Model file for the job. Use its own axes, mm. A direction names the side the tool comes from. Coordinates: 2 decimals unless noted, no trailing zeros. Order: outer loops, then holes, each group sorted by start corner. A loop starts at its lowest first (then second) coordinate and runs counter-clockwise, first axis right, second up. Notation, with made-up numbers: (41, 38) -> (63, 38) arc R27 cw to (63, 60) -> close; hole circle Ø10 at (42, 89.5). An arc over 180 degrees is marked (long way). Return JSON: item names as keys, results as strings. Group by question number.
1) Cut at D-D (x = -10). Write the cut outline in (y, z), and give its area (3 significant figures).
2) Probe line 1 (Y direction, x = 0, z = -1); line 2 (Y direction, x = 27.5, z = -1); line 3 (Y direction, x = 18.5, z = 3.5). List the from-to ranges inside material, lowest first.
3) Which spindle directions (+Z, -Z, +X, -X, +Y, -Y) get a long thin tool onto all of the face, cutting with end or side? Do faces 4 (the conical face through (-0.17, -4.13, -5.69)), 5 (the flat face through (0, 4.8, 0)). Say none if no direction does.
4) Cut at A-A (x = 0). Write the cut outline in (y, z).
5) Cut at B-B (z = 1.5). Write the cut outline in (x, y), and give its area (3 significant figures).
6) Pull direction Y, two halves, no side cores. Call faces 1 (the conical face through (-0.17, -4.12, 5.68)), 2 (the cylindrical face through (-6.607, -29.755, 0.089)), 3 (the flat face through (6, 0, -6.35)): +Y half, -Y half, draft (parallel to the pull), parting line (faces both ways), or undercut.
7) Cut at C-C (y = 0). Write the cut outline in (x, z), and give its area (3 significant figures).
8) Flat gauge pins, fed straight in: pin 1 (2 mm diameter, centred on x = 0.5, z = -3, fed in from -Y); pin 2 (2 mm diameter, centred on x = 8, z = -1, fed in from +Y); pin 3 (5 mm diameter, centred on y = 12, z = 5, fed in from +X). Where does each tip first touch, or does it go through?
from build123d import *

# Parameters (mm, degrees)
SKETCH1_R          = 30.48
SKETCH1_R_2        = 4
EXTRUDE1_DEPTH     = 6.35
CHAMFER1_SIZE      = 0.79375
SKETCH3_W          = 2
SKETCH3_H          = 2
CUT_EXTRUDE1_DEPTH = 45.937187273


with BuildPart() as part:
    # Sketch1 → Extrude1 (new, symmetric)
    with BuildSketch(Plane.XY):
        Circle(SKETCH1_R)
        Circle(SKETCH1_R_2, mode=Mode.SUBTRACT)
    extrude(amount=EXTRUDE1_DEPTH, both=True)

    # Chamfer1
    chamfer1_edges = [part.edges().sort_by_distance(p)[0] for p in [
        (-4, 0, -6.35),
        (-4, 0, 6.35),
    ]]
    chamfer(chamfer1_edges, length=CHAMFER1_SIZE)

    # Sketch3 → Cut-Extrude1 (cut, through all)
    with BuildSketch(Plane.XY.offset(6.35)):
        with Locations((0, 3.8)):
            Rectangle(SKETCH3_W, SKETCH3_H)
    extrude(amount=-CUT_EXTRUDE1_DEPTH, mode=Mode.SUBTRACT)


solid = part.part
Answers below:
{
 "1": {"outline": "(-28.79, -6.35) -> (28.79, -6.35) -> (28.79, 6.35) -> (-28.79, 6.35) -> close", "area": "731 mm^2"},
 "2": {"line 1": "y = -30.48 to -4, 4.8 to 30.48", "line 2": "y = -13.14 to 13.14", "line 3": "y = -24.22 to 24.22"},
 "3": {"face 4": "-Z", "face 5": "+Z, -Z"},
 "4": {"outline": "(-30.48, -6.35) -> (-4.79, -6.35) -> (-4, -5.56) -> (-4, 5.56) -> (-4.79, 6.35) -> (-30.48, 6.35) -> close; (4.8, -6.35) -> (30.48, -6.35) -> (30.48, 6.35) -> (4.8, 6.35) -> close"},
 "5": {"outline": "circle Ø60.96 at (0, 0); hole (-1, 3.87) arc R4 ccw (long way) to (1, 3.87) -> (1, 4.8) -> (-1, 4.8) -> close", "area": "2,870 mm^2"},
 "6": {"face 1": "undercut", "face 2": "parting line", "face 3": "draft"},
 "7": {"outline": "(-30.48, -6.35) -> (-4.79, -6.35) -> (-4, -5.56) -> (-4, 5.56) -> (-4.79, 6.35) -> (-30.48, 6.35) -> close; (4, -5.56) -> (4.79, -6.35) -> (30.48, -6.35) -> (30.48, 6.35) -> (4.79, 6.35) -> (4, 5.56) -> close", "area": "671 mm^2"},
 "8": {"pin 1": "stops at y = -30.48", "pin 2": "stops at y = 29.67", "pin 3": "stops at x = 28.96"}
}
